from build123d import *

# Parameters (mm, degrees)
SKETCH1_W           = 56.6674
SKETCH1_H           = 44.45
BOSS_EXTRUDE1_DEPTH = 1.5875
SKETCH2_W           = 43.6118
SKETCH2_H           = 39.3319
SKETCH2_W_2         = 41.0718
SKETCH2_H_2         = 36.7919
BOSS_EXTRUDE2_DEPTH = 2.54
SKETCH3_R           = 1.651
CUT_EXTRUDE1_DEPTH  = 37.099872308
SKETCH4_W           = 56.6674
SKETCH4_H           = 44.45
SKETCH4_W_2         = 55.6514
SKETCH4_H_2         = 43.434
CUT_EXTRUDE2_DEPTH  = 37.099872308
FILLET1_R           = 2.54
SKETCH5_W           = 12.7
SKETCH5_H           = 9.525
CUT_EXTRUDE3_DEPTH  = 36.388547151
CHAMFER1_SIZE       = 2.54


with BuildPart() as part:
    # Sketch1 → Boss-Extrude1 (new body)
    with BuildSketch(Plane(origin=(0, 0, 0), x_dir=(1, 0, 0), z_dir=(0, 1, 0))):
        Rectangle(SKETCH1_W, SKETCH1_H)
    extrude(amount=BOSS_EXTRUDE1_DEPTH)

    # Sketch2 → Boss-Extrude2 (add)
    with BuildSketch(Plane(origin=(0, 1.5875, 0), x_dir=(1, 0, 0), z_dir=(0, 1, 0))):
        with Locations((0, 0.79375)):
            Rectangle(SKETCH2_W, SKETCH2_H)
        with Locations((0, 0.79375)):
            Rectangle(SKETCH2_W_2, SKETCH2_H_2, mode=Mode.SUBTRACT)
    extrude(amount=BOSS_EXTRUDE2_DEPTH)

    # Sketch3 → Cut-Extrude1 (cut, through all)
    with BuildSketch(Plane(origin=(0, 1.5875, 0), x_dir=(1, 0, 0), z_dir=(0, 1, 0))):
        with Locations(Location((-24.5237, 0, 0), (0, 0, 270))):
            Circle(SKETCH3_R)
        with Locations(Location((24.5237, 0, 0), (0, 0, 270))):
            Circle(SKETCH3_R)
    extrude(amount=-CUT_EXTRUDE1_DEPTH, mode=Mode.SUBTRACT)

    # Sketch4 → Cut-Extrude2 (cut, through all)
    with BuildSketch(Plane(origin=(0, 1.5875, 0), x_dir=(1, 0, 0), z_dir=(0, 1, 0))):
        Rectangle(SKETCH4_W, SKETCH4_H)
        Rectangle(SKETCH4_W_2, SKETCH4_H_2, mode=Mode.SUBTRACT)
    extrude(amount=-CUT_EXTRUDE2_DEPTH, mode=Mode.SUBTRACT)

    # Fillet1
    fillet1_edges = [part.edges().sort_by_distance(p)[0] for p in [
        (27.8257, 0.79375, 21.717),
        (-27.8257, 0.79375, 21.717),
        (-27.8257, 0.79375, -21.717),
        (27.8257, 0.79375, -21.717),
    ]]
    fillet(fillet1_edges, radius=FILLET1_R)

    # Sketch5 → Cut-Extrude3 (cut, through all)
    with BuildSketch(Plane(origin=(0, 1.5875, 0), x_dir=(1, 0, 0), z_dir=(0, 1, 0))):
        with Locations((-15.4559, 15.6972)):
            Rectangle(SKETCH5_W, SKETCH5_H)
        with Locations((-15.4559, -14.1097)):
            Rectangle(SKETCH5_W, SKETCH5_H)
        with Locations((15.4559, -14.1097)):
            Rectangle(SKETCH5_W, SKETCH5_H)
        with Locations((15.4559, 15.6972)):
            Rectangle(SKETCH5_W, SKETCH5_H)
    extrude(amount=CUT_EXTRUDE3_DEPTH, mode=Mode.SUBTRACT)

    # Chamfer1
    chamfer1_edges = [part.edges().sort_by_distance(p)[0] for p in [
        (0, 1.5875, 17.6022),
        (20.5359, 1.5875, -0.79375),
        (0, 1.5875, -19.1897),
        (-20.5359, 1.5875, -0.79375),
    ]]
    chamfer(chamfer1_edges, length=CHAMFER1_SIZE - 0.0001)  # a hair under: the kernel refuses the full size


solid = part.part
The listing builds one solid part. Answer for the finished solid, in the listing's coordinates (mm). A direction names the side the tool comes from. Round coordinates to 2 decimals unless told otherwise and drop trailing zeros. Write each loop counter-clockwise with the first axis right and the second up, starting at its lowest first coordinate (ties: lowest second). Pieces come first, ordered by that corner, then holes. Notation, with made-up numbers: (-23.5, 32.5) - (-17.5, 32.5) arc R14 ccw to (-17.5, 50.5) - close; hole circle Ø5 at (21, 50). An arc over 180 degrees is marked (long way). Use a Markdown table: item, result. Add a question column.
1. The part is cut by section A-A (z = 0). Give the number of separate pieces and of enclosed holes in the cut face, and give its area (3 significant figures).
2. Flat-ended cylindrical pins translate along their axes: P1, Ø2, axis at x = 14.5, z = 16, coming from the +Y side; P2, Ø5.5, axis at x = -24.52, z = 0, coming from the +Y side; P3, Ø2, axis at y = 3, z = -18.5, coming from the +X side; P4, Ø0.8, axis at x = 19.5, y = 3, coming from the +Z side. Find the tip coordinate at first contact, or state that the pin passes through.
3. A tool of negligible diameter and unlimited length cuts with its end or side. For faces 5 (the face through (20, 3, 9.347)), 6 (the face through (9.106, 3, -19)), 7 (the face through (-20, 3, -10.935)), 8 (the face through (-9.106, 3, 17)), 9 (the face through (-27.101, 0.783, 20.953)), from which of +Z, -Z, +X, -X, +Y, -Y can it reach the whole face along a straight path? Write none if from no direction.
4. The part is cut by section C-C (y = 3.3). Write down the section's boundary in (x, z).
5. Consider line 1 (X direction, y = 0.7, z = 0); line 2 (Y direction, x = 7, z = -4.5); line 3 (Z direction, x = 8.5, y = 3.3). Determine where each line is inside the solid, lowest interval first.
6. For a pull along X with two mould halves and no side action, classify faces 1 (the face through (-0.13, 2.88, -17.94)), 2 (the face through (-27.826, 1, 0)), 3 (the face through (0, 1.588, 0)), 4 (the face through (27.101, 0.783, 20.953)) as +X half, -X half, draft (parallel to the pull), parting line (faces both ways), or undercut.
Reported:
| question | item | result |
|---|---|---|
| 1 | separate pieces | 3 |
| 1 | enclosed holes | 0 |
| 1 | area | 90.8 mm^2 |
| 2 | P1 | y = 1.59 |
| 2 | P2 | y = 4.13 |
| 2 | P3 | x = 9.11 |
| 2 | P4 | z = 9.35 |
| 3 | face 5 | +Z, +X, -X, +Y |
| 3 | face 6 | +Z, -Z, +X, +Y |
| 3 | face 7 | -Z, +X, -X, +Y |
| 3 | face 8 | +Z, -Z, -X, +Y |
| 3 | face 9 | +Z, -X, +Y, -Y |
| 4 | outline | (-21.81, -10.93) - (-19.71, -10.93) - (-19.71, 9.35) - (-21.81, 9.35) - close; (-9.11, -20.46) - (9.11, -20.46) - (9.11, -18.36) - (-9.11, -18.36) - close; (-9.11, 16.77) - (9.11, 16.77) - (9.11, 18.87) - (-9.11, 18.87) - close; (19.71, -10.93) - (21.81, -10.93) - (21.81, 9.35) - (19.71, 9.35) - close |
| 5 | line 1 | -27.83 to -26.17, -22.87 to 22.87, 26.17 to 27.83 |
| 5 | line 2 | 0 to 1.59 |
| 5 | line 3 | -20.46 to -18.36, 16.77 to 18.87 |
| 6 | face 1 | draft |
| 6 | face 2 | -X half |
| 6 | face 3 | undercut |
| 6 | face 4 | +X half |
